Geometry: see drawing. Coordinates: mm, zero at the bounding-box minimum. A direction names the side the tool comes from. Coordinates: 2 decimals unless noted, no trailing zeros. Loops run counter-clockwise (first coordinate to the right, second up) from the corner with the lowest first, then second, coordinate; pieces in that order, holes last. Notation, with made-up numbers: (-4, 11.5) -> (46, 11.5) arc R18 cw to (46, 18.5) -> close; hole circle Ø4 at (87.25, 45). An arc over 180 degrees is marked (long way). One line per item, written item: value. Start each with the question number.
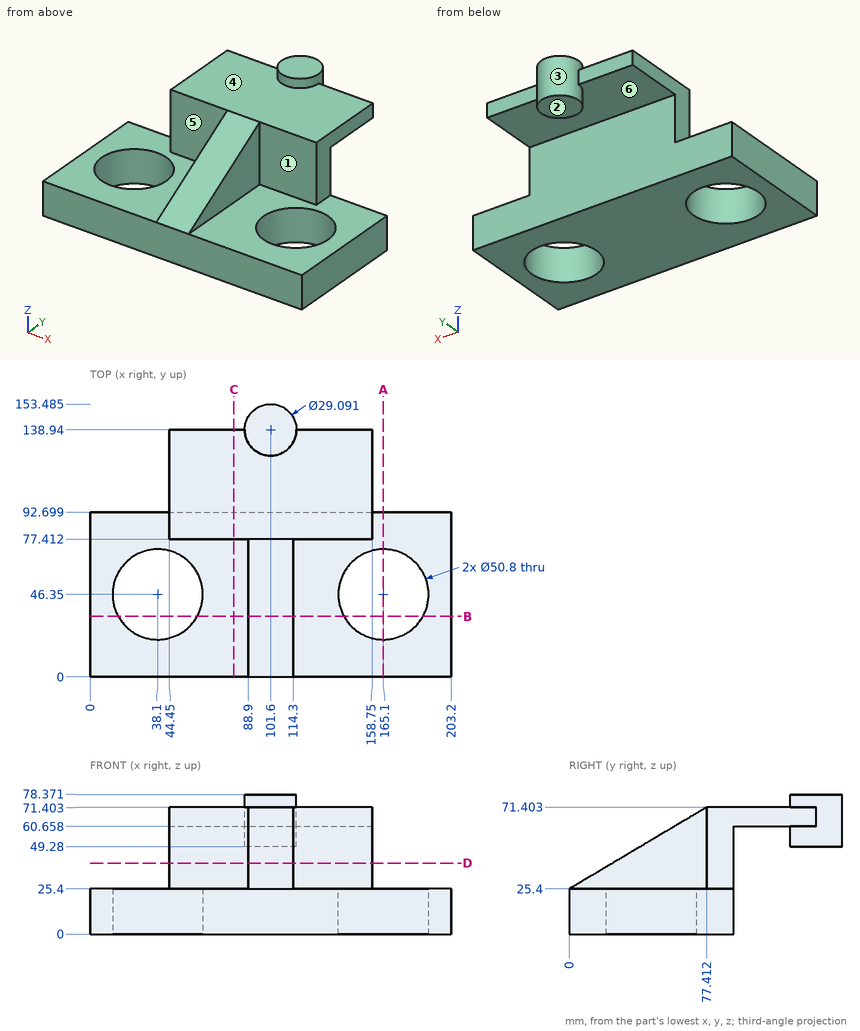
1. Draft query along Y for the marked faces 4, 5 and 6. Return one class per face: released by +Y, released by -Y, zero draft, split by the parting line, or undercut.
2. Set-up query: the marked faces 1, 2 and 3. Return all of +Z, -Z, +X, -X, +Y, -Y with unobstructed straight access to the full face (end or side cutting, diameter ignored); none if empty.
3. Section A-A on x = 165.1. Return the cut outline in (y, z), plus the area to 3 significant figures.
4. Section D-D on z = 40. Return the cut outline in (x, y), plus the area to 3 significant figures.
5. Section C-C on x = 81. Return the cut outline in (y, z).
6. Pin query (flat end, axial travel): pin 1 Ø3 at (x, z) = (133, 63.5) entering from +Y; pin 2 Ø1.5 at (y, z) = (77, 28) entering from +X; pin 3 Ø13.5 at (x, z) = (69, 47) entering from -Y; pin 4 Ø3 at (x, y) = (154, 68.5) entering from -Z. Return the tip coordinate at first contact, or that it passes through.
7. Line query: L1, parallel to Y at x = 165, z = 11; L2, parallel to X at y = 48.5, z = 19.5; L3, parallel to X at y = 92, z = 67.5. Output: solid intervals per line, ascending. Write a range as [from, to].
8. Section B-B on y = 34. Return the cut outline in (x, z) (1 decimal), plus the area to 3 significant figures.
Checks:
1. face 4: zero draft
1. face 5: released by -Y
1. face 6: undercut
2. face 1: +Z, +X, -Y
2. face 2: -Z, +X, -X, +Y
2. face 3: none
3. outline: (0, 0) -> (20.95, 0) -> (20.95, 25.4) -> (0, 25.4) -> close; (71.75, 0) -> (92.7, 0) -> (92.7, 25.4) -> (71.75, 25.4) -> close
3. area: 1,060 mm²
4. outline: (44.45, 77.41) -> (88.9, 77.41) -> (88.9, 24.57) -> (114.3, 24.57) -> (114.3, 77.41) -> (158.75, 77.41) -> (158.75, 92.7) -> (44.45, 92.7) -> close
4. area: 3,090 mm²
5. outline: (0, 0) -> (92.7, 0) -> (92.7, 60.66) -> (138.94, 60.66) -> (138.94, 71.4) -> (77.41, 71.4) -> (77.41, 25.4) -> (0, 25.4) -> close
6. pin 1: y = 138.94
6. pin 2: x = 158.75
6. pin 3: y = 77.41
6. pin 4: z = 0
7. L1: [0, 20.95], [71.75, 92.7]
7. L2: [0, 12.79], [63.41, 139.79], [190.41, 203.2]
7. L3: [44.45, 158.75]
8. outline: (0, 0) -> (15.9, 0) -> (15.9, 25.4) -> (0, 25.4) -> close; (60.3, 0) -> (142.9, 0) -> (142.9, 25.4) -> (114.3, 25.4) -> (114.3, 45.6) -> (88.9, 45.6) -> (88.9, 25.4) -> (60.3, 25.4) -> close; (187.3, 0) -> (203.2, 0) -> (203.2, 25.4) -> (187.3, 25.4) -> close
8. area: 3,420 mm²
